Here's how the part is built. I have some questions about the finished solid (model axes, mm). Face numbers are marked on the shaded views. A direction names the side the tool comes from. Give positions to 0.01 mm unless a question says otherwise; leave off trailing zeros. Order: outer loops, then holes, each group sorted by start corner. A loop starts at its lowest first (then second) coordinate and runs counter-clockwise, first axis right, second up. Notation, with made-up numbers: M 88,-3.75 L 112,-3.75 A21 ccw 112,20.25 Z; hole C -39.75,15 d10. An arc over 180 degrees is marked long. Use CSV: the item, a comma, the result in double quotes. Start each with the question number.
```python
from build123d import *

# Parameters (mm, degrees)
ESQUISSE1_R      = 5
EXTRUSION1_DEPTH = 3
ESQUISSE2_R      = 2
EXTRUSION2_DEPTH = 6
ESQUISSE3_R      = 2
EXTRUSION3_DEPTH = 2
ESQUISSE4_R      = 5
EXTRUSION4_DEPTH = 1
ESQUISSE5_W      = 6
ESQUISSE5_H      = 12
EXTRUSION5_DEPTH = 10
ESQUISSE6_W      = 3
ESQUISSE6_H      = 2
EXTRUSION6_DEPTH = 5


with BuildPart() as part:
    # Esquisse1 → Extrusion1 (new body)
    with BuildSketch(Plane(origin=(0, 0, 0), x_dir=(1, 0, 0), z_dir=(0, 1, 0))):
        Circle(ESQUISSE1_R)
    extrude(amount=EXTRUSION1_DEPTH)

    # Esquisse2 → Extrusion2 (add)
    with BuildSketch(Plane(origin=(0, 3, 0), x_dir=(-1, 0, 0), z_dir=(0, 1, 0))):
        Circle(ESQUISSE2_R)
    extrude(amount=EXTRUSION2_DEPTH)

    # Esquisse3 → Extrusion3 (add)
    with BuildSketch(Plane.XZ):
        Circle(ESQUISSE3_R)
    extrude(amount=EXTRUSION3_DEPTH)

    # Esquisse4 → Extrusion4 (add)
    with BuildSketch(Plane.XZ.offset(2)):
        Circle(ESQUISSE4_R)
    extrude(amount=EXTRUSION4_DEPTH)

    # Esquisse5 → Extrusion5 (add)
    with BuildSketch(Plane.XZ.offset(3)):
        Rectangle(ESQUISSE5_W, ESQUISSE5_H)
    extrude(amount=EXTRUSION5_DEPTH)

    # Esquisse6 → Extrusion6 (add)
    with BuildSketch(Plane.XZ.offset(13)):
        with Locations((0, 4)):
            Rectangle(ESQUISSE6_W, ESQUISSE6_H)
        Rectangle(ESQUISSE6_W, ESQUISSE6_H)
        with Locations((0, -4)):
            Rectangle(ESQUISSE6_W, ESQUISSE6_H)
    extrude(amount=EXTRUSION6_DEPTH)


solid = part.part
```
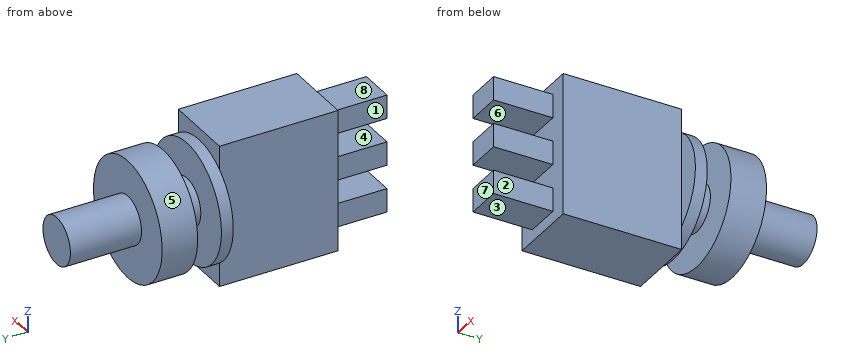
Q1. I need wall thicknesses on line 1 (Y direction, x = -4.5, z = 2); line 2 (Y direction, x = 1.25, z = -4.75); line 3 (X direction, y = -8.75, z = 2.5). Which ranges of each line are inside material? Lowest first, please. Write a range as [from, to].
Q2. Imagine slicing it at D-D, the plane z = 0. Please give me the cut outline in (x, y).
Q3. For the marked faces 1, 2, 3, 4 and 5, which set-ups out of +Z, -Z, +X, -X, +Y, -Y let a thin tool reach every point of the face, with its end or its side?
Q4. For P1, Ø5, axis at x = -1, z = 2.5, coming from the +Y side; P2, Ø1.5, axis at x = -0.5, y = -14.5, coming from the +Z side; P3, Ø2, axis at y = -15, z = 0, coming from the +X side; P4, Ø5, axis at y = -9, z = 2.5, coming from the +X side, each with a flat end and sliding along its axis, tell me the tip position at first contact or that it passes through.
Q5. We'd pull the mould along Z, two halves only. Please class the marked faces 6, 7 and 8: pulls with the +Z half, pulls with the -Z half, needs draft (parallel to the pull), parting line crosses it, or undercut.
Q6. Imagine slicing it at B-B, the plane z = 3.5. Please give me the cut outline in (x, y), then the cut area to 3 significant figures.
Q7. Imagine slicing it at A-A, the plane x = 2.75. Please give me the cut outline in (y, z), then the cut area to 3 significant figures.
Reply:
1,line 1,"y = [-3, -2], [0, 3]"
1,line 2,"y = [-18, -2], [0, 3]"
1,line 3,"x = [-3, 3]"
2,outline,"M -5,-3 L -3,-3 L -3,-13 L -1.5,-13 L -1.5,-18 L 1.5,-18 L 1.5,-13 L 3,-13 L 3,-3 L 5,-3 L 5,-2 L 2,-2 L 2,0 L 5,0 L 5,3 L 2,3 L 2,9 L -2,9 L -2,3 L -5,3 L -5,0 L -2,0 L -2,-2 L -5,-2 Z"
3,face 1,"+Z, -Z, -X, -Y"
3,face 2,"+Z, -Z, +X, -Y"
3,face 3,"-Z, +X, -X, -Y"
3,face 4,"+X, -X, -Y"
3,face 5,"+Y"
4,P1,"stops at y = 9"
4,P2,"stops at z = 5"
4,P3,"stops at x = 1.5"
4,P4,"stops at x = 3"
5,face 6,"undercut"
5,face 7,"needs draft"
5,face 8,"pulls with the +Z half"
6,outline,"M -3.57,-3 L -3,-3 L -3,-13 L -1.5,-13 L -1.5,-18 L 1.5,-18 L 1.5,-13 L 3,-13 L 3,-3 L 3.57,-3 L 3.57,-2 L -3.57,-2 Z; M -3.57,0 L 3.57,0 L 3.57,3 L -3.57,3 Z"
6,area,"104 mm^2"
7,outline,"M -13,-6 L -3,-6 L -3,-4.18 L -2,-4.18 L -2,4.18 L -3,4.18 L -3,6 L -13,6 Z; M 0,-4.18 L 3,-4.18 L 3,4.18 L 0,4.18 Z"
7,area,"153 mm^2"
